```python
from build123d import *

# Parameters (mm, degrees)
SKETCH_R           = 3.5
PAD_DEPTH          = 2
SKETCH001_W        = 4
SKETCH001_H        = 1.5
PAD001_DEPTH       = 7
POLARPATTERN_COUNT = 4


with BuildPart() as part:
    # Sketch → Pad (new body)
    with BuildSketch(Plane.XY):
        with BuildLine():
            Line((-8, 2), (-8, -2))
            Line((-8, -2), (-4.5, -2))
            ThreePointArc((-4.5, -2), (-3.482097, -3.482097), (-2, -4.5))
            Line((-2, -8), (-2, -4.5))
            Line((-2, -8), (2, -8))
            Line((2, -8), (2, -4.5))
            ThreePointArc((2, -4.5), (3.482097, -3.482097), (4.5, -2))
            Line((8, -2), (4.5, -2))
            Line((8, -2), (8, 2))
            Line((8, 2), (4.5, 2))
            ThreePointArc((4.5, 2), (3.482097, 3.482097), (2, 4.5))
            Line((2, 8), (2, 4.5))
            Line((2, 8), (-2, 8))
            Line((-2, 8), (-2, 4.5))
            ThreePointArc((-2, 4.5), (-3.482097, 3.482097), (-4.5, 2))
            Line((-8, 2), (-4.5, 2))
        make_face()
        Circle(SKETCH_R, mode=Mode.SUBTRACT)
    extrude(amount=-PAD_DEPTH)

    # Sketch001 → Pad001 (join)
    with BuildSketch(Plane.XY):
        with Locations((0, 7.25)):
            Rectangle(SKETCH001_W, SKETCH001_H)
    pad001 = extrude(amount=PAD001_DEPTH)

    # PolarPattern: Pad001 ×4 about axis
    polarpattern_axis = Axis((0, 0, 0), (0, 0, 1))
    for i in range(1, POLARPATTERN_COUNT):
        add(pad001.rotate(polarpattern_axis, i * 360 / POLARPATTERN_COUNT))


solid = part.part
```
Could you check a few things on this model? Use its own coordinates, in mm. A direction names the side the tool comes from. Give positions to 0.01 mm unless a question says otherwise; leave off trailing zeros. Loops run counter-clockwise (first coordinate to the right, second up) from the corner with the lowest first, then second, coordinate; pieces in that order, holes last. Notation, with made-up numbers: (24, 81.5) - (73, 81.5) arc R11 cw to (73, 92.5) - close; hole circle Ø8 at (-19, 42). An arc over 180 degrees is marked (long way). Answer in a Markdown table with one row per item. Add a question column.
Q1. If we section it at B-B (y = 0): List the corners of the cut face in (x, z) for me, plus the area to 3 significant figures.
Q2. If we section it at D-D (z = 5.75): List the corners of the cut face in (x, y) for me, plus the area to 3 significant figures.
Q3. Please list where these lines run through material, in increasing order: L1, parallel to X at y = -0.25, z = 0.75; L2, parallel to Y at x = 0, z = -0.35. Write a range as from..to.
Q4. Which directions (+Z, -Z, +X, -X, +Y, -Y) give clear straight access to the entire face, cutting with the end or side of a thin tool? Please do faces 1 (the face through (7, 2, 1)), 2 (the face through (-7, -2, 1)), 3 (the face through (7, -2, 1)), 4 (the face through (-2, 7, 1)), 5 (the face through (-6.5, 0, 3)).
Q5. We'd pull the mould along Y, two halves only. Please class faces 6 (the face through (1.4, 3.4, 0)), 7 (the face through (3.5, 3.464, -0.986)), 8 (the face through (8, 0, 2)): +Y half, -Y half, draft (parallel to the pull), parting line (faces both ways), or undercut.
Q6. If we section it at A-A (z = -0.5): List the corners of the cut face in (x, y) for me.
Q7. For pin 1 (3 mm diameter, centred on x = -2.5, y = -5.5, fed in from +Z); pin 2 (1.5 mm diameter, centred on x = 4.5, z = -0.5, fed in from -Y); pin 3 (6.5 mm diameter, centred on x = 0, y = 0, fed in from +Z); pin 4 (1 mm diameter, centred on y = 6.5, z = 1.5, fed in from +X), each with a flat end and sliding along its axis, tell me the tip position at first contact or that it passes through.
The answers:
| question | item | result |
|---|---|---|
| 1 | outline | (-8, -2) - (-3.5, -2) - (-3.5, 0) - (-6.5, 0) - (-6.5, 7) - (-8, 7) - close; (3.5, -2) - (8, -2) - (8, 7) - (6.5, 7) - (6.5, 0) - (3.5, 0) - close |
| 1 | area | 39.0 mm^2 |
| 2 | outline | (-8, -2) - (-6.5, -2) - (-6.5, 2) - (-8, 2) - close; (-2, -8) - (2, -8) - (2, -6.5) - (-2, -6.5) - close; (-2, 6.5) - (2, 6.5) - (2, 8) - (-2, 8) - close; (6.5, -2) - (8, -2) - (8, 2) - (6.5, 2) - close |
| 2 | area | 24.0 mm^2 |
| 3 | L1 | x = -8..-6.5, 6.5..8 |
| 3 | L2 | y = -8..-3.5, 3.5..8 |
| 4 | face 1 | +Z, -Z, +X, +Y |
| 4 | face 2 | +Z, -Z, -X, -Y |
| 4 | face 3 | +Z, -Z, +X, -Y |
| 4 | face 4 | +Z, -Z, -X, +Y |
| 4 | face 5 | +Z, +Y, -Y |
| 5 | face 6 | undercut |
| 5 | face 7 | +Y half |
| 5 | face 8 | draft |
| 6 | outline | (-8, -2) - (-4.5, -2) arc R4.92 ccw to (-2, -4.5) - (-2, -8) - (2, -8) - (2, -4.5) arc R4.92 ccw to (4.5, -2) - (8, -2) - (8, 2) - (4.5, 2) arc R4.92 ccw to (2, 4.5) - (2, 8) - (-2, 8) - (-2, 4.5) arc R4.92 ccw to (-4.5, 2) - (-8, 2) - close; hole circle Ø7 at (0, 0) |
| 7 | pin 1 | stops at z = 7 |
| 7 | pin 2 | stops at y = -3.19 |
| 7 | pin 3 | passes through |
| 7 | pin 4 | stops at x = 2 |
